from build123d import *

# Parameters (mm, degrees)
SKETCH_1_W          = 66
SKETCH_1_H          = 38
SKETCH_1_R          = 1.75
EXTRUDE_1_DEPTH     = 5
SKETCH_2_R          = 3.4
CUT_EXTRUDE_1_DEPTH = 3
SKETCH_3_W          = 1.5
SKETCH_3_H          = 1.5
CUT_EXTRUDE_2_DEPTH = 73
SKETCH_4_W          = 10
SKETCH_4_H          = 1.5
SKETCH_4_W_2        = 20
CUT_EXTRUDE_3_DEPTH = 1.5
FILLET_1_R          = 5
SKETCH_5_W          = 13
SKETCH_5_H          = 1.5
CUT_EXTRUDE_4_DEPTH = 1.5
SKETCH_6_W          = 20
SKETCH_6_H          = 10
SKETCH_6_W_2        = 10
CUT_EXTRUDE_5_DEPTH = 11.5
FILLET_2_R          = 2
SKETCH_7_W          = 10
SKETCH_7_H          = 2
SKETCH_7_W_2        = 20
EXTRUDE_2_DEPTH     = 5
SKETCH_8_W          = 10
SKETCH_8_H          = 2
SKETCH_8_W_2        = 20
CUT_EXTRUDE_6_DEPTH = 1.5
FILLET_3_R          = 2
SCALE_1_SCALE       = 0.6


with BuildPart() as part:
    # 草图1 → 凸台-拉伸1 (new body)
    with BuildSketch(Plane.XY):
        Rectangle(SKETCH_1_W, SKETCH_1_H)
        with Locations((-15, 0)):
            Circle(SKETCH_1_R, mode=Mode.SUBTRACT)
        with Locations(Location((15, 0, 0), (0, 0, 180))):
            Circle(SKETCH_1_R, mode=Mode.SUBTRACT)
    extrude(amount=EXTRUDE_1_DEPTH)

    # 草图2 → 切除-拉伸1 (cut)
    with BuildSketch(Plane.XY.offset(5)):
        with Locations((-15, 0)):
            Circle(SKETCH_2_R)
        with Locations((15, 0)):
            Circle(SKETCH_2_R)
    extrude(amount=-CUT_EXTRUDE_1_DEPTH, mode=Mode.SUBTRACT)

    # 草图3 → 切除-拉伸2 (cut)
    with BuildSketch(Plane.ZY.offset(33)):
        with Locations((4.25, 16.25)):
            Rectangle(SKETCH_3_W, SKETCH_3_H)
        with Locations((4.25, 13.25)):
            Rectangle(SKETCH_3_W, SKETCH_3_H)
        with Locations((4.25, 10.25)):
            Rectangle(SKETCH_3_W, SKETCH_3_H)
        with Locations((4.25, -10.25)):
            Rectangle(SKETCH_3_W, SKETCH_3_H)
        with Locations((4.25, -13.25)):
            Rectangle(SKETCH_3_W, SKETCH_3_H)
        with Locations((4.25, -16.25)):
            Rectangle(SKETCH_3_W, SKETCH_3_H)
    extrude(amount=-CUT_EXTRUDE_2_DEPTH, mode=Mode.SUBTRACT)

    # 草图4 → 切除-拉伸3 (cut)
    with BuildSketch(Plane.XY.offset(5)):
        with Locations((-28, 7.25)):
            Rectangle(SKETCH_4_W, SKETCH_4_H)
        with Locations((-28, -7.25)):
            Rectangle(SKETCH_4_W, SKETCH_4_H)
        with Locations((0, 7.25)):
            Rectangle(SKETCH_4_W_2, SKETCH_4_H)
        with Locations((0, -7.25)):
            Rectangle(SKETCH_4_W_2, SKETCH_4_H)
        with Locations((28, -7.25)):
            Rectangle(SKETCH_4_W, SKETCH_4_H)
        with Locations((28, 7.25)):
            Rectangle(SKETCH_4_W, SKETCH_4_H)
    extrude(amount=-CUT_EXTRUDE_3_DEPTH, mode=Mode.SUBTRACT)

    # 圆角1
    fillet_1_edges = [part.edges().sort_by_distance(p)[0] for p in [
        (33, -19, 2.5),
        (-33, -19, 2.5),
        (33, 19, 2.5),
        (-33, 19, 2.5),
    ]]
    fillet(fillet_1_edges, radius=FILLET_1_R - 0.0001)  # a hair under: the kernel refuses the full size

    # 草图5 → 切除-拉伸4 (cut)
    with BuildSketch(Plane.XY.offset(5)):
        with Locations((-16.5, 7.25)):
            Rectangle(SKETCH_5_W, SKETCH_5_H)
        with Locations((16.5, 7.25)):
            Rectangle(SKETCH_5_W, SKETCH_5_H)
        with Locations((-16.5, -7.25)):
            Rectangle(SKETCH_5_W, SKETCH_5_H)
        with Locations((16.5, -7.25)):
            Rectangle(SKETCH_5_W, SKETCH_5_H)
    extrude(amount=-CUT_EXTRUDE_4_DEPTH, mode=Mode.SUBTRACT)

    # 草图6 → 切除-拉伸5 (cut)
    with BuildSketch(Plane.XY.offset(5)):
        Rectangle(SKETCH_6_W, SKETCH_6_H)
        with Locations((25, 0)):
            Rectangle(SKETCH_6_W_2, SKETCH_6_H)
        with Locations((-25, 0)):
            Rectangle(SKETCH_6_W_2, SKETCH_6_H)
    extrude(amount=-CUT_EXTRUDE_5_DEPTH, mode=Mode.SUBTRACT)

    # 圆角2
    fillet_2_edges = [part.edges().sort_by_distance(p)[0] for p in [
        (-30, 5, 2.5),
        (-20, 5, 2.5),
        (-20, -5, 2.5),
        (-30, -5, 2.5),
        (20, -5, 2.5),
        (20, 5, 2.5),
        (30, 5, 2.5),
        (30, -5, 2.5),
        (-10, -5, 2.5),
        (-10, 5, 2.5),
        (10, 5, 2.5),
        (10, -5, 2.5),
    ]]
    fillet(fillet_2_edges, radius=FILLET_2_R)

    # 草图7 → 凸台-拉伸2 (add)
    with BuildSketch(Plane.XY.offset(5)):
        with Locations((-25, 0)):
            Rectangle(SKETCH_7_W, SKETCH_7_H)
        Rectangle(SKETCH_7_W_2, SKETCH_7_H)
        with Locations((25, 0)):
            Rectangle(SKETCH_7_W, SKETCH_7_H)
    extrude(amount=-EXTRUDE_2_DEPTH)

    # 草图8 → 切除-拉伸6 (cut)
    with BuildSketch(Plane.XY.offset(5)):
        with Locations((-25, 0)):
            Rectangle(SKETCH_8_W, SKETCH_8_H)
        Rectangle(SKETCH_8_W_2, SKETCH_8_H)
        with Locations((25, 0)):
            Rectangle(SKETCH_8_W, SKETCH_8_H)
    extrude(amount=-CUT_EXTRUDE_6_DEPTH, mode=Mode.SUBTRACT)

    # 圆角3
    fillet_3_edges = [part.edges().sort_by_distance(p)[0] for p in [
        (30, -1, 1.75),
        (30, 1, 1.75),
        (20, -1, 1.75),
        (20, 1, 1.75),
        (10, -1, 1.75),
        (10, 1, 1.75),
        (-10, -1, 1.75),
        (-10, 1, 1.75),
        (-30, -1, 1.75),
        (-20, -1, 1.75),
        (-20, 1, 1.75),
        (-30, 1, 1.75),
    ]]
    fillet(fillet_3_edges, radius=FILLET_3_R - 0.0001)  # a hair under: the kernel refuses the full size


with BuildPart() as part_1:
    # 缩放比例1: scaled about (0, 0, 0)
    add(part.part.scale(SCALE_1_SCALE))


solid = part_1.part
Build history of the part. All positions in model axes, mm. A direction names the side the tool comes from. Give positions to 0.01 mm unless a question says otherwise; leave off trailing zeros. Write item = value, one per line. Start each with the question number.
1) Band-saw the part on A-A on y = 0. Count the separate pieces of the cut face and the enclosed holes in it, plus the area to 3 significant figures.
2) Pull direction Y, two halves, no side cores. Call faces 4 (the cylindrical face through (12.361, -2.658, 1.479)), 5 (the cylindrical face through (18.9, 10.54, 1.52)), 6 (the flat face through (0, 5, 3)): +Y half, -Y half, draft (parallel to the pull), parting line (faces both ways), or undercut.
3) Tool access for faces 1 (the flat face through (-0.3, -7.5, 2.5)), 2 (the cylindrical face through (-17.639, -2.658, 1.479)), 3 (the flat face through (12, 0, 2.6)): list every direction of +Z, -Z, +X, -X, +Y, -Y with a clear straight run to the whole face (end or side of a thin tool).
4) Drop flat-ended pins along their axis: pin 1 Ø0.5 at (x, y) = (8.5, -8) entering from +Z; pin 2 Ø3.5 at (x, y) = (9, 0) entering from -Z. Give the stop position or say it passes through.
5) Probe probe 1 along Y at (x, z) = (-1.5, 0.5); probe 2 along Y at (x, z) = (-9, 2.05); probe 3 along Y at (x, z) = (17.5, 1.45). List the from-to ranges inside material, lowest first. Write a range as from..to.
Final values:
q1.separate_pieces = 3
q1.enclosed_holes = 0
q1.area = 77.5 mm²
q2.face_4 = undercut
q2.face_5 = +Y half
q2.face_6 = draft
q3.face_1 = +Z, +X, -X
q3.face_2 = +Z, -Z
q3.face_3 = +Z
q4.pin_1 = 2.1
q4.pin_2 = 0
q5.probe_1 = -11.4..-3, -0.6..0.6, 3..11.4
q5.probe_2 = -11.4..-2.04, 2.04..11.4
q5.probe_3 = -11.32..-2.77, -0.83..0.83, 2.77..11.32
